For this review, use the dimensioned drawing (mm, ordinates from the lowest corner) and the shaded views. A direction names the side the tool comes from. Give positions to 0.01 mm unless a question says otherwise; leave off trailing zeros. Loops run counter-clockwise (first coordinate to the right, second up) from the corner with the lowest first, then second, coordinate; pieces in that order, holes last. Notation, with made-up numbers: M 2,-3 L 8,-3 A18 cw 8,24 Z; hole C 42.5,35.5 d2. An arc over 180 degrees is marked long. Return JSON: item names as keys, results as strings.
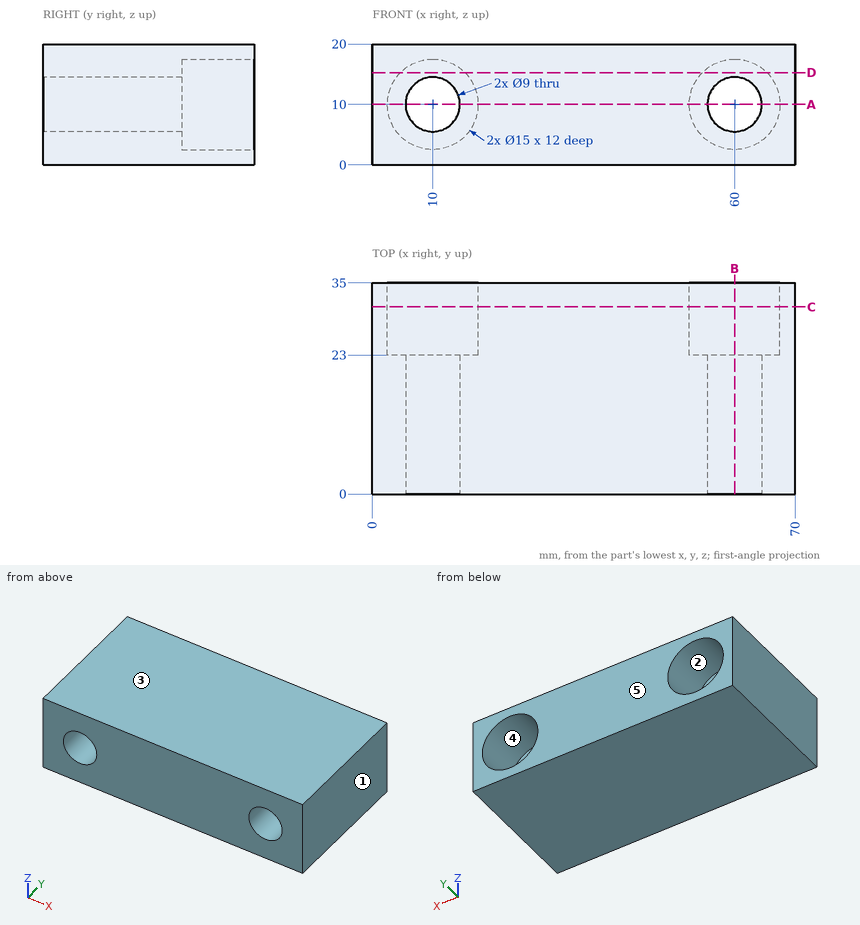
1) Consider section C-C on y = 31. Write out the cut boundary in (x, z), then the cut area to 3 significant figures.
From the geometry:
{"outline": "M 0,0 L 70,0 L 70,20 L 0,20 Z; hole C 10,10 d15; hole C 60,10 d15", "area": "1,050 mm²"}
2) The part is to be moulded in two halves that separate along X. For the marked faces 1, 2 and 3, say which applies: released by +X, released by -X, zero draft, split by the parting line, or undercut.
From the geometry:
{"face 1": "released by +X", "face 2": "undercut", "face 3": "zero draft"}
3) Consider section A-A on z = 10. Write out the cut boundary in (x, y), then the cut area to 3 significant figures.
From the geometry:
{"outline": "M 0,0 L 5.5,0 L 5.5,23 L 2.5,23 L 2.5,35 L 0,35 Z; M 14.5,0 L 55.5,0 L 55.5,23 L 52.5,23 L 52.5,35 L 17.5,35 L 17.5,23 L 14.5,23 Z; M 64.5,0 L 70,0 L 70,35 L 67.5,35 L 67.5,23 L 64.5,23 Z", "area": "1,680 mm²"}
4) Wall thickness on L1, parallel to X at y = 7, z = 10; L2, parallel to X at y = 28, z = 10; L3, parallel to Y at x = 9.5, z = 15.25: over which ranges is each line inside the solid? List them lowest first. Write a range as from..to.
From the geometry:
{"L1": "0..5.5, 14.5..55.5, 64.5..70", "L2": "0..2.5, 17.5..52.5, 67.5..70", "L3": "0..23"}
5) Consider section D-D on z = 15.25. Write out the cut boundary in (x, y), then the cut area to 3 significant figures.
From the geometry:
{"outline": "M 0,0 L 70,0 L 70,35 L 65.36,35 L 65.36,23 L 54.64,23 L 54.64,35 L 15.36,35 L 15.36,23 L 4.64,23 L 4.64,35 L 0,35 Z", "area": "2,190 mm²"}
6) Consider section B-B on x = 60. Write out the cut boundary in (y, z).
From the geometry:
{"outline": "M 0,0 L 35,0 L 35,2.5 L 23,2.5 L 23,5.5 L 0,5.5 Z; M 0,14.5 L 23,14.5 L 23,17.5 L 35,17.5 L 35,20 L 0,20 Z"}
7) Insertion check: pin 1 (4.5 mm diameter, centred on x = 7, z = 6.5, fed in from +Y); pin 2 (3 mm diameter, centred on x = 28, z = 16.5, fed in from -Y). Each pin has a flat end and moves straight along its axis. Give the tip position at first contact, or say it passes through.
From the geometry:
{"pin 1": "y = 23", "pin 2": "y = 0"}
8) Tool access review of the marked faces 4 and 5: name each direction out of +Z, -Z, +X, -X, +Y, -Y from which nothing blocks a thin tool from reaching the whole face with its end or side.
From the geometry:
{"face 4": "+Y", "face 5": "+Z, -Z, +X, -X, +Y"}
